Can you work these out from the model? Positions are in its coordinate system, mm. A direction names the side the tool comes from. Coordinates: 2 decimals unless noted, no trailing zeros. Order: outer loops, then holes, each group sorted by start corner. A loop starts at its lowest first (then second) coordinate and runs counter-clockwise, first axis right, second up. Notation, with made-up numbers: M 1,64 L 59,64 A5 ccw 59,69 Z; hole C 27,4 d10. An arc over 180 degrees is marked long. Answer as a JSON object with one key per item and string values.
from build123d import *

# Parameters (mm, degrees)
BOSS_EXTRUDE1_DEPTH = 152.4
SKETCH3_R           = 2.585
CUT_EXTRUDE1_DEPTH  = 167.951873679
CUT_EXTRUDE2_DEPTH  = 169.125169145
SKETCH5_R           = 3.175
CUT_EXTRUDE3_DEPTH  = 169.125169145


with BuildPart() as part:
    # Sketch2 → Boss-Extrude1 (new, symmetric)
    with BuildSketch(Plane.XY):
        with BuildLine():
            Line((-31.75, -31.75), (31.75, -31.75))
            Line((31.75, -31.75), (31.75, 31.75))
            Line((31.75, 31.75), (30.1625, 31.75))
            ThreePointArc((30.1625, 31.75), (29.039967985, 31.285032015), (28.575, 30.1625))
            Line((28.575, 30.1625), (28.575, -22.225))
            ThreePointArc((28.575, -22.225), (26.715128061, -26.715128061), (22.225, -28.575))
            Line((22.225, -28.575), (-30.1625, -28.575))
            ThreePointArc((-30.1625, -28.575), (-31.285032015, -29.039967985), (-31.75, -30.1625))
            Line((-31.75, -30.1625), (-31.75, -31.75))
        make_face()
    extrude(amount=BOSS_EXTRUDE1_DEPTH, both=True)

    # Sketch3 → Cut-Extrude1 (cut, through all)
    with BuildSketch(Plane(origin=(0, -28.575, 0), x_dir=(1, 0, 0), z_dir=(0, 1, 0))):
        with Locations(Location((-14.321922022, 8.79, 0), (0, 0, 180))):
            Circle(SKETCH3_R)
        with Locations(Location((6.678077978, 8.79, 0), (0, 0, 180))):
            Circle(SKETCH3_R)
        with Locations(Location((-14.321922022, 36.79, 0), (0, 0, 180))):
            Circle(SKETCH3_R)
        with Locations(Location((6.678077978, 36.79, 0), (0, 0, 180))):
            Circle(SKETCH3_R)
        with Locations(Location((-14.321922022, -36.79, 0), (0, 0, 180))):
            Circle(SKETCH3_R)
        with Locations(Location((6.678077978, -36.79, 0), (0, 0, 180))):
            Circle(SKETCH3_R)
        with Locations(Location((6.678077978, -8.79, 0), (0, 0, 180))):
            Circle(SKETCH3_R)
        with Locations(Location((-14.321922022, -8.79, 0), (0, 0, 180))):
            Circle(SKETCH3_R)
    extrude(amount=-CUT_EXTRUDE1_DEPTH, mode=Mode.SUBTRACT)

    # Sketch4 → Cut-Extrude2 (cut, through all)
    with BuildSketch(Plane(origin=(31.75, 0, 0), x_dir=(0, 0, -1), z_dir=(1, 0, 0))):
        Polygon((-152.4, 0), (-44, 0), (-44, -48.044655534), (-168.625421563, -48.044655534), (-168.625421563, 0), align=None)
        Polygon((168.625421563, -48.044655534), (168.625421563, 0), (152.4, 0), (44, 0), (44, -48.044655534), align=None)
    extrude(amount=-CUT_EXTRUDE2_DEPTH, mode=Mode.SUBTRACT)

    # Sketch5 → Cut-Extrude3 (cut, through all)
    with BuildSketch(Plane(origin=(31.75, 0, 0), x_dir=(0, 0, -1), z_dir=(1, 0, 0))):
        with Locations(Location((-44, 17.904243602, 0), (0, 0, 90))):
            Circle(SKETCH5_R)
        with Locations(Location((44, 17.904243602, 0), (0, 0, 90))):
            Circle(SKETCH5_R)
    extrude(amount=-CUT_EXTRUDE3_DEPTH, mode=Mode.SUBTRACT)


solid = part.part
Item 1: If we mould it in two halves opening along Z, with no side actions, what happens to faces 1 (the flat face through (-4, -28.575, 1)), 2 (the flat face through (7, -29, 44)), 3 (the cylindrical face through (5.485, -30.14, -11.083))? For each: pulls with the +Z half, pulls with the -Z half, needs draft (parallel to the pull), parting line crosses it, or undercut.
Answers follow:
{"face 1": "needs draft", "face 2": "pulls with the +Z half", "face 3": "undercut"}
Item 2: I want a section at C-C, the plane y = -4. Write out the boundary of the cut face in (x, z) (3 decimals).
Answers follow:
{"outline": "M 28.575,-44 L 31.75,-44 L 31.75,44 L 28.575,44 Z"}
Item 3: I'm going to push flat-ended pins straight in: pin 1 (15.5 mm diameter, centred on x = 1, z = -19.5, fed in from +Y) (3 decimals); pin 2 (8.5 mm diameter, centred on y = 17.9, z = -44, fed in from -X) (3 decimals); pin 3 (1.6 mm diameter, centred on x = 30, z = 106.5, fed in from -Y). Where does each tip first touch, or does it pass through?
Answers follow:
{"pin 1": "stops at y = -28.575", "pin 2": "stops at x = 28.575", "pin 3": "stops at y = 0"}
Item 4: I want a section at D-D, the plane x = -9. Write out the boundary of the cut face in (y, z) (3 decimals), plus the area to 3 significant figures.
Answers follow:
{"outline": "M -31.75,-44 L -28.575,-44 L -28.575,44 L -31.75,44 Z", "area": "279 mm^2"}
Item 5: Which directions (+Z, -Z, +X, -X, +Y, -Y) give clear straight access to the entire face, cutting with the end or side of a thin tool? Please do faces 4 (the flat face through (7, -29, -44)), 5 (the cylindrical face through (30.18, 17.22, 40.9)), 6 (the flat face through (28.575, 10, 2)).
Answers follow:
{"face 4": "-Z, +X, -X, -Y", "face 5": "+X, -X", "face 6": "+Z, -Z, -X, +Y"}
Item 6: I want a section at A-A, the plane z = 36.79. Give the number of separate pieces and of enclosed holes in the cut face, plus the area to 3 significant figures.
Answers follow:
{"separate pieces": "3", "enclosed holes": "0", "area": "368 mm^2"}
Item 7: Please list where these lines run through material, in increasing order: line 1 (X direction, y = 20.5, z = 13.5) (3 decimals); line 2 (X direction, y = -30, z = 8); line 3 (X direction, y = -29, z = -8).
Answers follow:
{"line 1": "x = 28.575 to 31.75", "line 2": "x = -31.74 to -16.78, -11.86 to 4.22, 9.14 to 31.75", "line 3": "x = -31.24 to -16.78, -11.86 to 4.22, 9.14 to 31.75"}
